```python
from build123d import *

# Parameters (mm, degrees)
RESSALTO_EXTRUS_O1_DEPTH = 10
FILETE1_R                = 2
FILETE2_R                = 2
RESSALTO_EXTRUS_O2_DEPTH = 26
FILETE4_R                = 2
FILETE6_R                = 2


with BuildPart() as part:
    # Esboço1 → Ressalto-extrusão1 (new body)
    with BuildSketch(Plane.XY):
        Polygon((-17.957860615883305, -18.6871961102107), (-2.9578606158833054, -18.687196110210696), (-2.957860615883306, -13.687196110210696), (-2.957860615883306, -8.687196110210698), (7.042139384116819, -8.687196110210696), (7.042139384116693, 11.312803889789302), (-17.95786061588331, 11.312803889789302), align=None)
        with BuildLine():
            Line((-2.957860615883306, -8.687196110210698), (-2.957860615883306, -13.687196110210696))
            ThreePointArc((-2.9578606158833054, -13.687196110210696), (1.451969440367277, -10.006856222711722), (7.042139384116818, -8.6871961102107))
            Line((7.042139384116819, -8.687196110210696), (-2.957860615883306, -8.687196110210698))
        make_face()
        Polygon((7.042139384116693, 11.312803889789302), (7.0421393841166955, -8.687196110210698), (17.042139384116695, -8.687196110210696), (17.042139384116698, -13.687196110210698), (17.042139384116698, -18.687196110210696), (32.042139384116695, -18.687196110210692), (32.042139384116695, 11.31280388978931), align=None)
        with BuildLine():
            Line((17.042139384116695, -8.687196110210696), (7.042139384116819, -8.687196110210696))
            ThreePointArc((7.042139384116818, -8.6871961102107), (12.632309327866226, -10.006856222711777), (17.0421393841167, -13.687196110210698))
            Line((17.042139384116698, -13.687196110210698), (17.042139384116695, -8.687196110210696))
        make_face()
    extrude(amount=RESSALTO_EXTRUS_O1_DEPTH)

    # Filete1
    filete1_edges = [part.edges().sort_by_distance(p)[0] for p in [
        (17.042139384116695, -16.187196110210696, 10),
        (17.042139384116695, -16.187196110210696, 0),
        (7.042139384116695, -8.6871961102107, 0),
        (-2.9578606158833054, -13.687196110210696, 5),
        (-2.9578606158833054, -18.6871961102107, 5),
        (17.042139384116695, -18.687196110210696, 5),
        (17.0421393841167, -13.687196110210698, 5),
        (-2.9578606158833054, -16.1871961102107, 10),
        (7.042139384116694, -8.6871961102107, 10),
        (-2.9578606158833054, -16.1871961102107, 0),
    ]]
    fillet(filete1_edges, radius=FILETE1_R)

    # Filete2
    filete2_edges = [part.edges().sort_by_distance(p)[0] for p in [
        (-17.957860615883305, -18.6871961102107, 5),
        (-17.95786061588331, 11.312803889789302, 5),
        (32.042139384116695, 11.31280388978931, 5),
        (32.042139384116695, -18.687196110210692, 5),
    ]]
    fillet(filete2_edges, radius=FILETE2_R)

    # Esboço2 → Ressalto-extrusão2 (add)
    with BuildSketch(Plane.XY.offset(10)):
        Polygon((9.042139384116691, 9.312803889789297), (5.042139384116695, 9.312803889789297), (5.042139384116695, 5.312803889789297), (-14.957860615883307, 5.312803889789293), (-14.957860615883302, -6.771146492865117), (-10.957860615883302, -6.771146492865116), (-10.957860615883309, 1.312803889789298), (5.042139384116695, 1.3128038897893), (5.042139384116695, -2.6871961102106985), (9.042139384116695, -2.687196110210697), (9.042139384116693, 1.3128038897892964), (25.04213938411669, 1.3128038897893024), (25.042139384116695, -6.771146492865112), (29.042139384116695, -6.771146492865111), (29.042139384116695, 5.312803889789296), (9.042139384116693, 5.312803889789297), align=None)
    extrude(amount=RESSALTO_EXTRUS_O2_DEPTH)

    # Filete4
    filete4_edges = [part.edges().sort_by_distance(p)[0] for p in [
        (-10.957860615883309, 1.312803889789298, 23),
        (25.042139384116695, 1.3128038897893024, 23),
    ]]
    fillet(filete4_edges, radius=FILETE4_R)

    # Filete6
    filete6_edges = [part.edges().sort_by_distance(p)[0] for p in [
        (-14.957860615883305, -0.729171301537912, 10),
        (27.042139384116695, -6.771146492865111, 10),
        (29.042139384116695, -0.7291713015379075, 10),
        (7.042139384116693, 9.312803889789297, 10),
        (5.042139384116695, 7.312803889789297, 10),
        (-4.957860615883305, 5.312803889789295, 10),
        (9.042139384116691, 7.312803889789297, 10),
        (19.042139384116695, 5.312803889789297, 10),
        (-12.957860615883302, -6.771146492865116, 10),
    ]]
    fillet(filete6_edges, radius=FILETE6_R - 0.0001)  # a hair under: the kernel refuses the full size


solid = part.part
```
The model under review builds one solid part; all positions refer to its coordinate system, in mm. A direction names the side the tool comes from. Coordinates: 2 decimals unless noted, no trailing zeros. Write each loop counter-clockwise with the first axis right and the second up, starting at its lowest first coordinate (ties: lowest second). Pieces come first, ordered by that corner, then holes.
1) The part is to be moulded in two halves that separate along X. For faces 5 (the face through (-10.4, 0.7, 23.2)), 6 (the face through (-13.25, -7.37, 10.57)), 7 (the face through (24.441, 0.742, 23.182)), 8 (the face through (29.644, -0.617, 10.57)), say which applies: pulls with the +X half, pulls with the -X half, needs draft (parallel to the pull), parting line crosses it, or undercut.
2) We need section C-C on z = 33. State the section outline as (x, y) points, then the cut area to 3 significant figures.
3) We need section D-D on z = 4.5. State the section outline as (x, y) points.
4) To check wall thickness, follow probe 1 along X at (y, z) = (-2.5, 23); probe 2 along X at (y, z) = (1, 13.5); probe 3 along Y at (x, z) = (-13, 25.5). State the ranges of each line that lie inside material, in increasing order.
5) Machinability: for faces 1 (the face through (9.042, -1, 23)), 2 (the face through (5.042, 7, 24)), 3 (the face through (-2.84, -13.71, 5.04)), 4 (the face through (9.644, 7.688, 10.57)), which of the approach directions +Z, -Z, +X, -X, +Y, -Y give a long, thin tool a straight path to every point of the face, cutting with its end or side? Answer none if there is none.
6) Clearance check with flat-ended pins moving along their axes: pin 1 Ø4.5 at (x, z) = (6.5, 20.5) entering from -Y; pin 2 Ø6.5 at (y, z) = (-3, 26) entering from -X; pin 3 Ø1.2 at (x, z) = (7, 23) entering from +Y. State where each tip first meets the part, or that it passes through.
7) We need section A-A on y = -1.5. State the section outline as (x, z) points.
8) We need section B-B on x = 21. State the section outline as (y, z) points, then the cut area to 3 significant figures.
Answer list:
1. face 5: undercut
1. face 6: needs draft
1. face 7: undercut
1. face 8: pulls with the +X half
2. outline: (-14.96, -6.77) - (-10.96, -6.77) - (-10.96, -0.69) arc R2 cw to (-8.96, 1.31) - (5.04, 1.31) - (5.04, -2.69) - (9.04, -2.69) - (9.04, 1.31) - (23.04, 1.31) arc R2 cw to (25.04, -0.69) - (25.04, -6.77) - (29.04, -6.77) - (29.04, 5.31) - (9.04, 5.31) - (9.04, 9.31) - (5.04, 9.31) - (5.04, 5.31) - (-14.96, 5.31) - close
2. area: 274 mm2
3. outline: (-17.96, -16.69) arc R2 ccw to (-15.96, -18.69) - (-4.96, -18.69) arc R2 ccw to (-2.96, -16.69) - (-2.96, -14.39) arc R2 cw to (-2.48, -13.09) arc R12.5 cw to (16.57, -13.09) arc R2 cw to (17.04, -14.39) - (17.04, -16.69) arc R2 ccw to (19.04, -18.69) - (30.04, -18.69) arc R2 ccw to (32.04, -16.69) - (32.04, 9.31) arc R2 ccw to (30.04, 11.31) - (-15.96, 11.31) arc R2 ccw to (-17.96, 9.31) - close
4. probe 1: x = -14.96 to -10.96, 5.04 to 9.04, 25.04 to 29.04
4. probe 2: x = -14.96 to -10.03, 5.04 to 9.04, 24.12 to 29.04
4. probe 3: y = -6.77 to 5.31
5. face 1: +Z, -Y
5. face 2: +Z, -X, +Y
5. face 3: +Z, -Z, -Y
5. face 4: +Z, +X, +Y
6. pin 1: stops at y = -2.69
6. pin 2: stops at x = -14.96
6. pin 3: stops at y = 9.31
7. outline: (-17.96, 0) - (32.04, 0) - (32.04, 10) - (31.04, 10) arc R2 cw to (29.04, 12) - (29.04, 36) - (25.04, 36) - (25.04, 10) - (9.04, 10) - (9.04, 36) - (5.04, 36) - (5.04, 10) - (-10.96, 10) - (-10.96, 36) - (-14.96, 36) - (-14.96, 12) arc R2 cw to (-16.96, 10) - (-17.96, 10) - close
8. outline: (-18.69, 0) - (11.31, 0) - (11.31, 10) - (7.31, 10) arc R2 cw to (5.31, 12) - (5.31, 36) - (1.31, 36) - (1.31, 10) - (-18.69, 10) - close
8. area: 405 mm2
